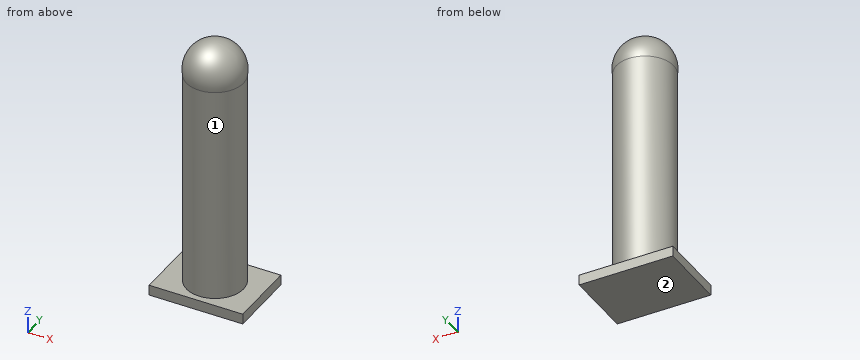
```python
from build123d import *

# Parameters (mm, degrees)
ESQUISSE1_W        = 27
ESQUISSE1_H        = 20
BOSS_EXTRU_1_DEPTH = 3
ESQUISSE2_R        = 8.23653306
BOSS_EXTRU_2_DEPTH = 63
D_ME1_FACE_RADIUS  = 8.23653306
D_ME1_HEIGHT       = 10


with BuildPart() as part:
    # Esquisse1 → Boss.-Extru.1 (new body)
    with BuildSketch(Plane.XY):
        with Locations((-32.019829949, 16.119881557)):
            Rectangle(ESQUISSE1_W, ESQUISSE1_H)
    extrude(amount=BOSS_EXTRU_1_DEPTH)

    # Esquisse2 → Boss.-Extru.2 (add)
    with BuildSketch(Plane.XY.offset(3)):
        with Locations((-32.019829949, 16.119881557)):
            Circle(ESQUISSE2_R)
    extrude(amount=BOSS_EXTRU_2_DEPTH)

    # Dôme1: a dome of height H over a round flat face of radius A is a cap of a sphere of radius (A * A + H * H) / (2 * H)
    d_me1_r = (D_ME1_FACE_RADIUS * D_ME1_FACE_RADIUS + D_ME1_HEIGHT * D_ME1_HEIGHT) / (2 * D_ME1_HEIGHT)
    d_me1_base = Plane((-32.019829949, 16.119881557, 66), z_dir=(0, 0, 1))
    with Locations(d_me1_base.offset(D_ME1_HEIGHT - d_me1_r)):
        d_me1_ball = Sphere(d_me1_r, mode=Mode.PRIVATE)
    add(split(d_me1_ball, bisect_by=d_me1_base, keep=Keep.TOP, mode=Mode.PRIVATE))


solid = part.part
```
For this review, take the finished solid that the model builds, in its own axes (mm). Face numbers are marked on the shaded views. Give positions to 0.01 mm unless a question says otherwise; leave off trailing zeros. Write each loop counter-clockwise with the first axis right and the second up, starting at its lowest first coordinate (ties: lowest second). Pieces come first, ordered by that corner, then holes. Notation, with made-up numbers: M 56,48 L 92,48 A24 cw 92,65 Z; hole C -6.5,58.5 d5. An arc over 180 degrees is marked long. One line per item, written item: value.
1) Take a section at A-A, the plane x = -39.25. Write out the cut boundary in (y, z).
Results are:
outline: M 6.12,0 L 26.12,0 L 26.12,3 L 20.07,3 L 20.07,66 A4.26 ccw long 12.17,66 L 12.17,3 L 6.12,3 Z
2) For P1, Ø5, axis at x = -28, z = 17.5, coming from the -Y side; P2, Ø2, axis at x = -29, y = 23, coming from the -Z side; P3, Ø5, axis at y = 15, z = 40.5, coming from the -X side; P4, Ø10, axis at x = -25, z = 49.5, coming from the +Y side, all flat-tipped, find the tip position at first contact; note any pin that passes through.
Results are:
P1: stops at y = 8.02
P2: stops at z = 0
P3: stops at x = -40.26
P4: stops at y = 24.1
3) For line 1 (Z direction, x = -23.5, y = 14); line 2 (Y direction, x = -32, z = 41); line 3 (Z direction, x = -31, y = 20.5), list the stretches that pass through material, from the lowest coordinate up. Write a range as from..to.
Results are:
line 1: z = 0..3
line 2: y = 7.88..24.36
line 3: z = 0..74.69
4) The part is to be moulded in two halves that separate along Z. For the marked faces 1 and 2, say which applies: +Z half, -Z half, draft (parallel to the pull), parting line (faces both ways), or undercut.
Results are:
face 1: undercut
face 2: -Z half
5) Take a section at D-D, the plane y = 25.25. Write out the cut boundary in (x, z), then the cut area to 3 significant figures.
Results are:
outline: M -45.52,0 L -18.52,0 L -18.52,3 L -45.52,3 Z
area: 81.0 mm²
6) Take a section at B-B, the plane y = 11. Write out the cut boundary in (x, z), then the cut area to 3 significant figures.
Results are:
outline: M -45.52,0 L -18.52,0 L -18.52,3 L -25.57,3 L -25.57,66 A6.65 ccw long -38.47,66 L -38.47,3 L -45.52,3 Z
area: 985 mm²
7) Take a section at C-C, the plane z = 10. Write out the cut boundary in (x, y).
Results are:
outline: C -32.02,16.12 d16.47
